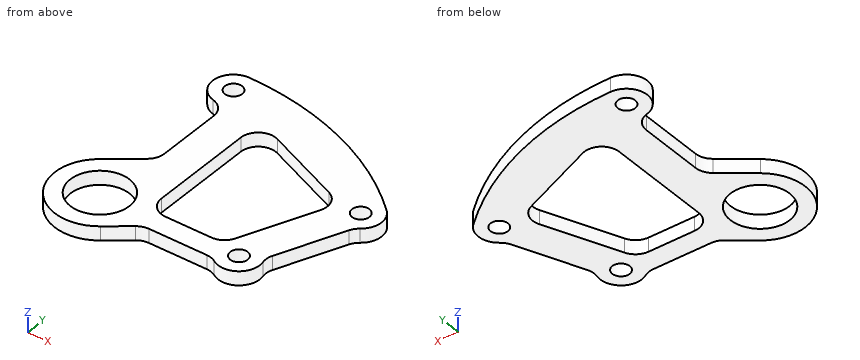
```python
from build123d import *

# Parameters (mm, degrees)
SKETCH1_R           = 17
SKETCH1_R_2         = 5
BOSS_EXTRUDE1_DEPTH = 4


with BuildPart() as part:
    # Sketch1 → Boss-Extrude1 (new, symmetric)
    with BuildSketch(Plane.XY):
        with BuildLine():
            Line((5, 78.575714714), (5, 41.77822761))
            ThreePointArc((5, 41.77822761), (3.987940463, 37.394516142), (1.156614753, 33.898120074))
            Line((1.156614753, 33.898120074), (-16.007198358, 20.488279594))
            ThreePointArc((-16.007198358, 20.488279594), (-20.488279594, -16.007198358), (16.007198358, -20.488279594))
            Line((16.007198358, -20.488279594), (28.65699687, -10.605173838))
            ThreePointArc((28.65699687, -10.605173838), (31.557930079, -9.030095618), (34.813611624, -8.485281374))
            Line((34.813611624, -8.485281374), (68.071279511, -8.485281374))
            ThreePointArc((68.071279511, -8.485281374), (70.897583966, -8.892992642), (73.493425188, -10.08288075))
            ThreePointArc((73.493425188, -10.08288075), (86.982957468, -9.759011477), (91.643297853, 2.904068715))
            ThreePointArc((91.643297853, 2.904068715), (91.376524695, 6.104282152), (92.137861813, 9.224041719))
            Line((92.137861813, 9.224041719), (107.806206108, 46.218943848))
            ThreePointArc((107.806206108, 46.218943848), (109.157818303, 48.505648792), (111.063780403, 50.355833512))
            ThreePointArc((111.063780403, 50.355833512), (115.90879124, 59.4152181), (111.968703818, 68.903225806))
            ThreePointArc((111.968703818, 68.903225806), (59.988170877, 100.853839718), (0, 112))
            ThreePointArc((0, 112), (-11.921234951, 101.372646075), (-2.727272727, 88.314026208))
            ThreePointArc((-2.727272727, 88.314026208), (2.833494518, 84.791530319), (5, 78.575714714))
        make_face()
        Circle(SKETCH1_R, mode=Mode.SUBTRACT)
        with Locations((0, 100)):
            Circle(SKETCH1_R_2, mode=Mode.SUBTRACT)
        with Locations((80, 0)):
            Circle(SKETCH1_R_2, mode=Mode.SUBTRACT)
        with Locations((103.923048454, 60)):
            Circle(SKETCH1_R_2, mode=Mode.SUBTRACT)
        with BuildLine():
            Line((25, 72.976113171), (25, 13.514718626))
            ThreePointArc((25, 13.514718626), (27.928932188, 6.443650814), (35, 3.514718626))
            Line((35, 3.514718626), (61.375366857, 3.514718626))
            ThreePointArc((61.375366857, 3.514718626), (66.898085507, 5.178077893), (70.583551108, 9.614802884))
            Line((70.583551108, 9.614802884), (88.006080219, 50.7515527))
            ThreePointArc((88.006080219, 50.7515527), (88.058512057, 58.42519202), (82.657599567, 63.876580264))
            Line((82.657599567, 63.876580264), (38.8597036, 82.201224993))
            ThreePointArc((38.8597036, 82.201224993), (29.459108194, 81.300686313), (25, 72.976113171))
        make_face(mode=Mode.SUBTRACT)
    extrude(amount=BOSS_EXTRUDE1_DEPTH, both=True)


solid = part.part
```
Geometry: final body of the model. Coordinates: model frame, mm. Give positions to 0.01 mm unless a question says otherwise; leave off trailing zeros. Order: outer loops, then holes, each group sorted by start corner. A loop starts at its lowest first (then second) coordinate and runs counter-clockwise, first axis right, second up. Notation, with made-up numbers: (39, 36.25) -> (98, 36.25) arc R9 cw to (98, 40.25) -> close; hole circle Ø2 at (-17.5, 66.25). An arc over 180 degrees is marked (long way). Write each question's results on one line, items separated by ' | '. Start each with the question number.
1) First-contact query: pin 1 (1 mm diameter, centred on y = 18.5, z = 2, fed in from -X); pin 2 (11.5 mm diameter, centred on x = 80, y = 0, fed in from -Z); pin 3 (10 mm diameter, centred on x = 88.5, y = 94, fed in from +Z); pin 4 (2.5 mm diameter, centred on y = 58.5, z = -1.5, fed in from -X). Flat tips, straight axial feed; report the tip coordinate or a pass-through.
2) Section A-A (y = 23). Return loops of the section in (x, z).
3) Section C-C (z = -1.25). Return loops of the section in (x, y), then the cut area to 3 significant figures.
4) Section D-D (y = 60). Return loops of the section in (x, z).
5) Section B-B (x = 80). Return loops of the section in (y, z).
6) Line query: line 1 (Y direction, x = 0, z = 1.5); line 2 (Y direction, x = 80, z = 0); line 3 (X direction, y = 15, z = 2.25). Output: solid intervals per line, ascending. Write a range as from..to.
Calculated:
1) pin 1: x = -18.76 | pin 2: z = -4 | pin 3: through | pin 4: x = 5
2) outline: (-12.79, -4) -> (25, -4) -> (25, 4) -> (-12.79, 4) -> close; (76.25, -4) -> (97.97, -4) -> (97.97, 4) -> (76.25, 4) -> close
3) outline: (-16.01, 20.49) arc R26 ccw to (16.01, -20.49) -> (28.66, -10.61) arc R10 cw to (34.81, -8.49) -> (68.07, -8.49) arc R10 cw to (73.49, -10.08) arc R12 ccw to (91.64, 2.9) arc R10 cw to (92.14, 9.22) -> (107.81, 46.22) arc R10 cw to (111.06, 50.36) arc R12 ccw to (111.97, 68.9) arc R167 ccw to (0, 112) arc R12 ccw to (-2.73, 88.31) arc R10 cw to (5, 78.58) -> (5, 41.78) arc R10 cw to (1.16, 33.9) -> close; hole circle Ø34 at (0, 0); hole circle Ø10 at (0, 100); hole (25, 13.51) arc R10 ccw to (35, 3.51) -> (61.38, 3.51) arc R10 ccw to (70.58, 9.61) -> (88.01, 50.75) arc R10 ccw to (82.66, 63.88) -> (38.86, 82.2) arc R10 ccw to (25, 72.98) -> close; hole circle Ø10 at (80, 0); hole circle Ø10 at (103.92, 60) | area: 7,590 mm2
4) outline: (5, -4) -> (25, -4) -> (25, 4) -> (5, 4) -> close; (87.25, -4) -> (98.92, -4) -> (98.92, 4) -> (87.25, 4) -> close; (108.92, -4) -> (115.92, -4) -> (115.92, 4) -> (108.92, 4) -> close
5) outline: (-12, -4) -> (-5, -4) -> (-5, 4) -> (-12, 4) -> close; (5, -4) -> (31.85, -4) -> (31.85, 4) -> (5, 4) -> close; (64.99, -4) -> (91.59, -4) -> (91.59, 4) -> (64.99, 4) -> close
6) line 1: -26..-17, 17..32.99, 87.24..95, 105..112 | line 2: -12..-5, 5..31.85, 64.99..91.59 | line 3: -21.24..-8, 8..25, 72.86..94.58
